CAD build for the part. Positions are in the model's coordinates, mm. A direction names the side the tool comes from. Round coordinates to 2 decimals unless told otherwise and drop trailing zeros. Loops run counter-clockwise (first coordinate to the right, second up) from the corner with the lowest first, then second, coordinate; pieces in that order, holes last.
```python
from build123d import *

# Parameters (mm, degrees)
SKETCH1_R           = 2.15
BOSS_EXTRUDE1_DEPTH = 40


with BuildPart() as part:
    # Sketch1 → Boss-Extrude1 (new body)
    with BuildSketch(Plane(origin=(0, 0, 0), x_dir=(-1, 0, 0), z_dir=(0, 0, -1))):
        with BuildLine():
            Line((-12.499999997, 0.800000003), (-12.499999998, 1.500000003))
            ThreePointArc((-12.499999998, 1.500000003), (-12.587867964, 1.712132039), (-12.8, 1.800000005))
            Line((-12.8, 1.800000005), (-14.9175884, 1.800000005))
            ThreePointArc((-14.9175884, 1.800000005), (-15.686636445, 2.313861481), (-15.506192291, 3.221015502))
            Line((-15.506192291, 3.221015502), (-13.255887451, 5.471320342))
            ThreePointArc((-13.255887451, 5.471320342), (-12.282617405, 6.121638595), (-11.134567109, 6.349999998))
            Line((-11.134567109, 6.349999998), (-8.865432906, 6.349999998))
            ThreePointArc((-8.865432906, 6.349999998), (-7.717382611, 6.121638596), (-6.744112565, 5.471320342))
            Line((-6.744112565, 5.471320342), (-4.493807727, 3.221015504))
            ThreePointArc((-4.493807727, 3.221015504), (-4.313363573, 2.313861481), (-5.082411619, 1.800000005))
            Line((-5.082411619, 1.800000005), (-7.20000001, 1.800000005))
            ThreePointArc((-7.20000001, 1.800000005), (-7.412132045, 1.71213204), (-7.50000001, 1.500000005))
            Line((-7.50000001, 1.500000005), (-7.50000001, 0.8))
            ThreePointArc((-7.50000001, 0.8), (-7.265685435, 0.234314575), (-6.70000001, 0))
            Line((-6.70000001, 0), (-2, 0))
            ThreePointArc((-2, 0), (-0.585786438, 0.585786438), (0, 2))
            Line((0, 2), (0, 6.699999998))
            ThreePointArc((0, 6.699999998), (-0.234314576, 7.265685424), (-0.800000003, 7.5))
            Line((-0.800000003, 7.5), (-1.500000007, 7.5))
            ThreePointArc((-1.500000007, 7.5), (-1.712132044, 7.412132033), (-1.80000001, 7.199999997))
            Line((-1.80000001, 7.199999997), (-1.80000001, 5.082411604))
            ThreePointArc((-1.80000001, 5.082411604), (-2.313861485, 4.313363559), (-3.221015507, 4.493807713))
            Line((-3.221015507, 4.493807713), (-5.471320347, 6.744112553))
            ThreePointArc((-5.471320347, 6.744112553), (-6.1216386, 7.717382599), (-6.350000003, 8.865432896))
            Line((-6.350000003, 8.865432896), (-6.350000003, 11.134567105))
            ThreePointArc((-6.350000003, 11.134567105), (-6.121638601, 12.2826174), (-5.471320347, 13.255887446))
            Line((-5.471320347, 13.255887446), (-3.221015511, 15.506192282))
            ThreePointArc((-3.221015511, 15.506192282), (-2.313861487, 15.686636436), (-1.80000001, 14.917588389))
            Line((-1.80000001, 14.917588389), (-1.80000001, 12.799999998))
            ThreePointArc((-1.80000001, 12.799999998), (-1.712132045, 12.587867963), (-1.50000001, 12.499999997))
            Line((-1.50000001, 12.499999997), (-0.8, 12.499999997))
            ThreePointArc((-0.8, 12.499999997), (-0.234314575, 12.734314573), (0, 13.299999998))
            Line((0, 13.299999998), (0, 18))
            ThreePointArc((0, 18), (-0.585786438, 19.414213562), (-2, 20))
            Line((-2, 20), (-6.700000008, 20))
            ThreePointArc((-6.700000008, 20), (-7.265685435, 19.765685424), (-7.50000001, 19.199999998))
            Line((-7.50000001, 19.199999998), (-7.50000001, 18.500000005))
            ThreePointArc((-7.50000001, 18.500000005), (-7.412132044, 18.287867969), (-7.200000008, 18.200000003))
            Line((-7.200000008, 18.200000003), (-5.082411595, 18.200000003))
            ThreePointArc((-5.082411595, 18.200000003), (-4.313363547, 17.686138525), (-4.493807702, 16.7789845))
            Line((-4.493807702, 16.7789845), (-6.744112543, 14.528679659))
            ThreePointArc((-6.744112543, 14.528679659), (-7.717382589, 13.878361405), (-8.865432885, 13.650000003))
            Line((-8.865432885, 13.650000003), (-11.134567111, 13.650000003))
            ThreePointArc((-11.134567111, 13.650000003), (-12.282617406, 13.878361405), (-13.255887452, 14.528679658))
            Line((-13.255887452, 14.528679658), (-15.506192292, 16.778984498))
            ThreePointArc((-15.506192292, 16.778984498), (-15.686636447, 17.686138525), (-14.917588397, 18.200000002))
            Line((-14.917588397, 18.200000002), (-12.799999998, 18.200000003))
            ThreePointArc((-12.799999998, 18.200000003), (-12.587867963, 18.287867968), (-12.499999997, 18.500000002))
            Line((-12.499999997, 18.500000002), (-12.499999997, 19.2))
            ThreePointArc((-12.499999997, 19.2), (-12.734314573, 19.765685425), (-13.299999998, 20))
            Line((-13.299999998, 20), (-18, 20))
            ThreePointArc((-18, 20), (-19.414213562, 19.414213562), (-20, 18))
            Line((-20, 18), (-20, 13.3))
            ThreePointArc((-20, 13.3), (-19.765685424, 12.734314573), (-19.199999998, 12.499999997))
            Line((-19.199999998, 12.499999997), (-18.500000003, 12.499999997))
            ThreePointArc((-18.500000003, 12.499999997), (-18.287867967, 12.587867964), (-18.2, 12.8))
            Line((-18.2, 12.8), (-18.2, 14.91758839))
            ThreePointArc((-18.2, 14.91758839), (-17.686138525, 15.686636435), (-16.778984504, 15.506192281))
            Line((-16.778984504, 15.506192281), (-14.528679657, 13.255887434))
            ThreePointArc((-14.528679657, 13.255887434), (-13.878361403, 12.282617388), (-13.65, 11.134567091))
            Line((-13.65, 11.134567091), (-13.65, 8.865432887))
            ThreePointArc((-13.65, 8.865432887), (-13.878361403, 7.717382591), (-14.528679656, 6.744112546))
            Line((-14.528679656, 6.744112546), (-16.778984496, 4.493807706))
            ThreePointArc((-16.778984496, 4.493807706), (-17.686138522, 4.313363551), (-18.2, 5.0824116))
            Line((-18.2, 5.0824116), (-18.2, 7.2))
            ThreePointArc((-18.2, 7.2), (-18.287867966, 7.412132034), (-18.5, 7.5))
            Line((-18.5, 7.5), (-19.2, 7.5))
            ThreePointArc((-19.2, 7.5), (-19.765685425, 7.265685425), (-20, 6.7))
            Line((-20, 6.7), (-20, 2))
            ThreePointArc((-20, 2), (-19.414213562, 0.585786438), (-18, 0))
            Line((-18, 0), (-13.3, 0))
            ThreePointArc((-13.3, 0), (-12.734314573, 0.234314576), (-12.499999997, 0.800000003))
        make_face()
        with Locations((-10, 10)):
            Circle(SKETCH1_R, mode=Mode.SUBTRACT)
    extrude(amount=-BOSS_EXTRUDE1_DEPTH)


solid = part.part
```
Item 1: Cut at A-A, the plane x = 10. Give the cut face in (y, z).
Answers follow:
outline: (6.35, 0) - (7.85, 0) - (7.85, 40) - (6.35, 40) - close; (12.15, 0) - (13.65, 0) - (13.65, 40) - (12.15, 40) - close
Item 2: Probe line 1 (Y direction, x = 10, z = 22); line 2 (X direction, y = 14.5, z = 35); line 3 (X direction, y = 5, z = 18.5). List the from-to ranges inside material, lowest first.
Answers follow:
line 1: y = 6.35 to 7.85, 12.15 to 13.65
line 2: x = 0 to 1.8, 4.23 to 6.77, 13.23 to 15.77, 18.2 to 20
line 3: x = 0 to 1.8, 3.73 to 6.27, 13.73 to 16.27, 18.2 to 20
Item 3: Flat gauge pins, fed straight in: P1, Ø0.7, axis at y = 9.5, z = 28.5, coming from the -X side; P2, Ø0.6, axis at y = 1.5, z = 25.5, coming from the +X side; P3, Ø0.8, axis at x = 1, z = 28.5, coming from the +Y side. Where does each tip first touch, or does it go through?
Answers follow:
P1: stops at x = 6.35
P2: stops at x = 19.99
P3: stops at y = 19.91
Item 4: Two-plate mould, pull along Y, no slides. Class faces 6 (the flat face through (20, 16, 20)), 7 (the flat face through (10, 6.35, 20)), 8 (the flat face through (18.2, 14, 20)), 9 (the cylindrical face through (19.4, 19.43, 19.72)): released by +Y, released by -Y, zero draft, split by the parting line, or undercut.
Answers follow:
face 6: zero draft
face 7: released by -Y
face 8: undercut
face 9: released by +Y
Item 5: 3-axis set-ups, long thin cutter, end or side, ignore diameter. For faces 1 (the cylindrical face through (13.872, 7.733, 19.72)), 2 (the cylindrical face through (19.77, 12.74, 19.72)), 3 (the cylindrical face through (12.74, 0.23, 19.72)), 4 (the flat face through (0, 16, 20)), 5 (the cylindrical face through (0.24, 12.73, 19.72)): which of +Z, -Z, +X, -X, +Y, -Y reach the whole face in a straight line?
Answers follow:
face 1: +Z, -Z
face 2: +Z, -Z, +X
face 3: +Z, -Z, -Y
face 4: +Z, -Z, -X, +Y, -Y
face 5: +Z, -Z, -X
